Build history of the part. All positions in model axes, mm. Face numbers are marked on the shaded views. A direction names the side the tool comes from. Give positions to 0.01 mm unless a question says otherwise; leave off trailing zeros. Order: outer loops, then holes, each group sorted by start corner. A loop starts at its lowest first (then second) coordinate and runs counter-clockwise, first axis right, second up. Notation, with made-up numbers: (79.25, 81) - (104.25, 81) arc R15 cw to (104.25, 90) - close; hole circle Ø2 at (-9.75, 0). An arc over 180 degrees is marked (long way). Answer in a Markdown table with one row per item.
```python
from build123d import *

# Parameters (mm, degrees)
SKETCH_1_W               = 17.5
SKETCH_1_H               = 55
EXTRUDE_1_DEPTH          = 2
SKETCH_2_W               = 5
SKETCH_2_H               = 5
EXTRUDE_2_DEPTH          = 33
EXTRUDE_3_DEPTH          = 6.5
EXTRUDE_3_DEPTH_BACK     = 8.378522314
SKETCH_3_W               = 5
SKETCH_3_H               = 55
SKETCH_4_R               = 1.5
CUT_EXTRUDE_1_DEPTH      = 10
FILLET_1_R               = 10
SKETCH_5_R               = 4
CUT_EXTRUDE_2_DEPTH      = 12
EXTRUDE_START            = -14.878522
EXTRUDE_4_DEPTH          = 14.878522
SKETCH_7_W               = 4
SKETCH_7_H               = 2
SKETCH_7_W_2             = 2.3
SKETCH_7_H_2             = 5.8
EXTRUDE_5_DEPTH          = 42.173435595
SKETCH_9_R               = 2
CUT_EXTRUDE_15_DEPTH     = 39
CUT_EXTRUDE_START        = -6.3
CUT_EXTRUDE_16_OUTLINE_W = 24
CUT_EXTRUDE_16_OUTLINE_H = 9.8
CUT_EXTRUDE_16_DEPTH     = 6.3


# Read off the part's stored shape, not the designer's step: Вырез-Вытянуть16
with BuildPart() as part:
    # Эскиз1 → Бобышка-Вытянуть1 (new body)
    with BuildSketch(Plane(origin=(0, 0, 0), x_dir=(1, 0, 0), z_dir=(0, 1, 0))):
        with Locations((8.75, 27.5)):
            Rectangle(SKETCH_1_W, SKETCH_1_H)
    extrude(amount=EXTRUDE_1_DEPTH)

    # Эскиз2 → Бобышка-Вытянуть2 (add)
    with BuildSketch(Plane(origin=(0, 2, 0), x_dir=(1, 0, 0), z_dir=(0, 1, 0))):
        with Locations((2.5, 52.5)):
            Rectangle(SKETCH_2_W, SKETCH_2_H)
        with Locations((2.5, 2.5)):
            Rectangle(SKETCH_2_W, SKETCH_2_H)
    extrude(amount=EXTRUDE_2_DEPTH)

    # Эскиз3 → Бобышка-Вытянуть3 (add, two sides: drawn at the far end of the back side and taken through both)
    with BuildSketch(Plane(origin=(0, 35, 0), x_dir=(1, 0, 0), z_dir=(0, 1, 0)).offset(-EXTRUDE_3_DEPTH_BACK)):
        with Locations((2.5, 27.5)):
            Rectangle(SKETCH_3_W, SKETCH_3_H)
    extrude(amount=EXTRUDE_3_DEPTH + EXTRUDE_3_DEPTH_BACK)

    # Эскиз4 → Вырез-Вытянуть1 (cut)
    with BuildSketch(Plane(origin=(0, 2, 0), x_dir=(1, 0, 0), z_dir=(0, 1, 0))):
        with Locations(Location((11.449842766, 48, 0), (0, 0, 270))):
            Circle(SKETCH_4_R)
        with Locations(Location((11.449842766, 7, 0), (0, 0, 270))):
            Circle(SKETCH_4_R)
    extrude(amount=-CUT_EXTRUDE_1_DEPTH, mode=Mode.SUBTRACT)

    # Скругление1
    # the kernel refuses this fillet: 10 mm, written as the material it adds along each edge
    with BuildSketch(Plane(origin=(5, 2, -50), x_dir=(0, 0, 1), z_dir=(-1, 0, 0)), Plane(origin=(5, 2, 0), x_dir=(0, 1, 0), z_dir=(0, 0, -1))) as fillet_1_piece_1:
        with BuildLine():
            CenterArc((FILLET_1_R, FILLET_1_R), FILLET_1_R, 180, 90)
            Line((0, FILLET_1_R), (0, 0))
            Line((0, 0), (FILLET_1_R, 0))
        make_face()
    extrude(amount=5)
    with BuildSketch(Plane(origin=(5, 2, -55), x_dir=(0, 1, 0), z_dir=(0, 0, 1)), Plane(origin=(5, 2, -5), x_dir=(0, 0, -1), z_dir=(-1, 0, 0))) as fillet_1_piece_2:
        with BuildLine():
            CenterArc((FILLET_1_R, -FILLET_1_R), FILLET_1_R, 90, 90)
            Line((0, -FILLET_1_R), (0, 0))
            Line((0, 0), (FILLET_1_R, 0))
        make_face()
    extrude(amount=5)
    with BuildSketch(Plane(origin=(5, 2, -55), x_dir=(0, 1, 0), z_dir=(0, 0, 1))) as fillet_1_piece_3a_section:
        with BuildLine():
            CenterArc((FILLET_1_R, -FILLET_1_R), FILLET_1_R, 90, 90)
            Line((0, -FILLET_1_R), (0, 0))
            Line((0, 0), (FILLET_1_R, 0))
        make_face()
    fillet_1_piece_3a = extrude(amount=30, mode=Mode.PRIVATE)
    fillet_1_piece_3a = split(fillet_1_piece_3a, bisect_by=Plane(origin=(7.224830191, 4.283537978, -50), z_dir=(0, 0, 1)), keep=Keep.TOP, mode=Mode.PRIVATE)
    fillet_1_piece_3a = fillet_1_piece_3a - Plane(origin=(11.449842766, 4.283537978, -48), x_dir=(0, 0, 1), z_dir=(0, 1, 0)) * Cylinder(1.5, 100, mode=Mode.PRIVATE)
    with BuildSketch(Plane(origin=(30, 2, -50), x_dir=(0, 0, 1), z_dir=(-1, 0, 0))) as fillet_1_piece_3b_section:
        with BuildLine():
            CenterArc((FILLET_1_R, FILLET_1_R), FILLET_1_R, 180, 90)
            Line((0, FILLET_1_R), (0, 0))
            Line((0, 0), (FILLET_1_R, 0))
        make_face()
    fillet_1_piece_3b = extrude(amount=30, mode=Mode.PRIVATE)
    fillet_1_piece_3b = split(fillet_1_piece_3b, bisect_by=Plane(origin=(5, 2.276950555, -42.605283247), z_dir=(1, 0, 0)), keep=Keep.TOP, mode=Mode.PRIVATE)
    fillet_1_piece_3b = split(fillet_1_piece_3b, bisect_by=Plane(origin=(17.5, 2.276950555, -42.605283247), z_dir=(-1, 0, 0)), keep=Keep.TOP, mode=Mode.PRIVATE)
    fillet_1_piece_3b = fillet_1_piece_3b - Plane(origin=(11.449842766, 2.276950555, -48), x_dir=(0, 0, 1), z_dir=(0, 1, 0)) * Cylinder(1.5, 100, mode=Mode.PRIVATE)
    fillet_1_piece_3 = fillet_1_piece_3a & fillet_1_piece_3b
    add(fillet_1_piece_3)
    with BuildSketch(Plane(origin=(5, 2, 0), x_dir=(0, 1, 0), z_dir=(0, 0, -1))) as fillet_1_piece_4a_section:
        with BuildLine():
            CenterArc((FILLET_1_R, FILLET_1_R), FILLET_1_R, 180, 90)
            Line((0, FILLET_1_R), (0, 0))
            Line((0, 0), (FILLET_1_R, 0))
        make_face()
    fillet_1_piece_4a = extrude(amount=30, mode=Mode.PRIVATE)
    fillet_1_piece_4a = split(fillet_1_piece_4a, bisect_by=Plane(origin=(7.224831151, 4.283537771, -5), z_dir=(0, 0, -1)), keep=Keep.TOP, mode=Mode.PRIVATE)
    fillet_1_piece_4a = fillet_1_piece_4a - Plane(origin=(11.449842766, 4.283537771, -7), x_dir=(0, 0, 1), z_dir=(0, 1, 0)) * Cylinder(1.5, 100, mode=Mode.PRIVATE)
    with BuildSketch(Plane(origin=(30, 2, -5), x_dir=(0, 0, -1), z_dir=(-1, 0, 0))) as fillet_1_piece_4b_section:
        with BuildLine():
            CenterArc((FILLET_1_R, -FILLET_1_R), FILLET_1_R, 90, 90)
            Line((0, -FILLET_1_R), (0, 0))
            Line((0, 0), (FILLET_1_R, 0))
        make_face()
    fillet_1_piece_4b = extrude(amount=30, mode=Mode.PRIVATE)
    fillet_1_piece_4b = split(fillet_1_piece_4b, bisect_by=Plane(origin=(5, 2.276949142, -12.394716375), z_dir=(1, 0, 0)), keep=Keep.TOP, mode=Mode.PRIVATE)
    fillet_1_piece_4b = split(fillet_1_piece_4b, bisect_by=Plane(origin=(17.5, 2.276949142, -12.394716375), z_dir=(-1, 0, 0)), keep=Keep.TOP, mode=Mode.PRIVATE)
    fillet_1_piece_4b = fillet_1_piece_4b - Plane(origin=(11.449842766, 2.276949142, -7), x_dir=(0, 0, 1), z_dir=(0, 1, 0)) * Cylinder(1.5, 100, mode=Mode.PRIVATE)
    fillet_1_piece_4 = fillet_1_piece_4a & fillet_1_piece_4b
    add(fillet_1_piece_4)

    # Эскиз5 → Вырез-Вытянуть2 (cut)
    with BuildSketch(Plane(origin=(0, 2, 0), x_dir=(1, 0, 0), z_dir=(0, 1, 0))):
        with Locations((11.449842766, 48)):
            Circle(SKETCH_5_R)
        with Locations((11.449842766, 7)):
            Circle(SKETCH_5_R)
    extrude(amount=CUT_EXTRUDE_2_DEPTH, mode=Mode.SUBTRACT)

    # Эскиз6 → Бобышка-Вытянуть4 (add)
    with BuildSketch(Plane(origin=(0, 41.5, 0), x_dir=(1, 0, 0), z_dir=(0, 1, 0)).offset(EXTRUDE_START)):
        with BuildLine():
            Line((0, 4.85), (0, 6.15))
            Line((0, 6.15), (-1.92, 6.15))
            Line((-1.92, 6.15), (-2.88, 4.487231225))
            ThreePointArc((-2.88, 4.487231225), (-2.642083488, 3.599314712), (-1.754166975, 3.837231225))
            Line((-1.754166975, 3.837231225), (-1.16944465, 4.85))
            Line((-1.16944465, 4.85), (0, 4.85))
        make_face()
        with BuildLine():
            Line((0, 28.65), (0, 29.95))
            Line((0, 29.95), (-1.16944465, 29.95))
            Line((-1.16944465, 29.95), (-1.754166975, 30.962768775))
            ThreePointArc((-1.754166975, 30.962768775), (-2.642083488, 31.200685288), (-2.88, 30.312768775))
            Line((-2.88, 30.312768775), (-1.92, 28.65))
            Line((-1.92, 28.65), (0, 28.65))
        make_face()
    extrude(amount=EXTRUDE_4_DEPTH)

    # Эскиз7 → Бобышка-Вытянуть5 (add)
    with BuildSketch(Plane.XY):
        with Locations((9.3, 40.5)):
            Rectangle(SKETCH_7_W, SKETCH_7_H)
        with Locations((6.15, 40.5)):
            Rectangle(SKETCH_7_W_2, SKETCH_7_H)
        with Locations((9.3, 36.6)):
            Rectangle(SKETCH_7_W, SKETCH_7_H_2)
        Polygon((7.3, 33.7), (5, 33.7), (5, 31.7), (11.3, 31.7), (11.3, 33.7), align=None)
    extrude(amount=-EXTRUDE_5_DEPTH)

    # Эскиз9 → Вырез-Вытянуть15 (cut)
    with BuildSketch(Plane(origin=(11.3, 0, 0), x_dir=(0, 0, -1), z_dir=(1, 0, 0))):
        with Locations((37, 36.5)):
            Circle(SKETCH_9_R)
        with Locations((5, 36.5)):
            Circle(SKETCH_9_R)
    extrude(amount=-CUT_EXTRUDE_15_DEPTH, mode=Mode.SUBTRACT)

    # Вырез-Вытянуть16 outline → Вырез-Вытянуть16 (cut)
    with BuildSketch(Plane(origin=(11.3, 0, 0), x_dir=(0, 0, -1), z_dir=(1, 0, 0)).offset(CUT_EXTRUDE_START)):
        with Locations((21, 36.6)):
            Rectangle(CUT_EXTRUDE_16_OUTLINE_W, CUT_EXTRUDE_16_OUTLINE_H)
    extrude(amount=CUT_EXTRUDE_16_DEPTH, mode=Mode.SUBTRACT)


solid = part.part
```
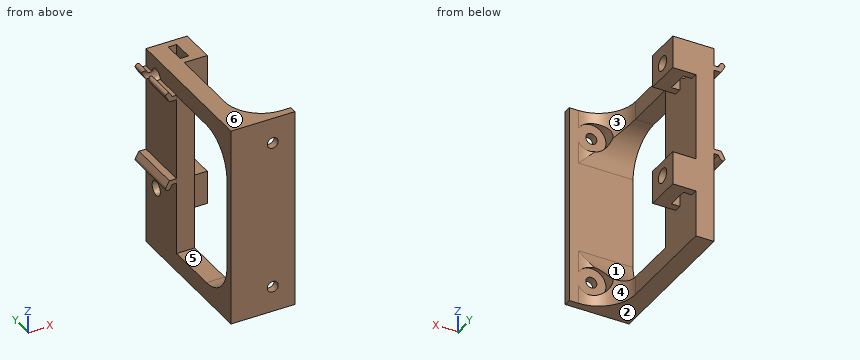
1. Cut at C-C on x = 2. Write the cut outline in (y, z).
Check result:
| item | result |
|---|---|
| outline | (0, -55) - (41.5, -55) - (41.5, 0) - (0, 0) - close; hole (2, -40) arc R10 ccw to (12, -50) - (26.62, -50) - (26.62, -5) - (12, -5) arc R10 ccw to (2, -15) - close; hole circle Ø4 at (36.5, -37); hole circle Ø4 at (36.5, -5) |
2. Cut at B-B on z = -25.5. Write the cut outline in (x, y).
Check result:
| item | result |
|---|---|
| outline | (0, 0) - (17.5, 0) - (17.5, 2) - (0, 2) - close; (0, 26.62) - (5, 26.62) - (5, 41.5) - (0, 41.5) - close |
3. Drop flat-ended pins along their axis: P1, Ø2, axis at x = -1.5, y = 31, coming from the -Z side; P2, Ø4, axis at y = 28, z = -16.5, coming from the +X side; P3, Ø3, axis at y = 35.5, z = -35.5, coming from the +X side; P4, Ø4, axis at y = 7, z = -45, coming from the +X side. Give the stop position or say it passes through.
Check result:
| item | result |
|---|---|
| P1 | stops at z = -31.29 |
| P2 | stops at x = 5 |
| P3 | stops at x = 11.3 |
| P4 | passes through |
4. Which spindle directions (+Z, -Z, +X, -X, +Y, -Y) get a long thin tool onto all of the face, cutting with end or side? Do the marked faces 1 and 2. Say none if no direction does.
Check result:
| item | result |
|---|---|
| face 1 | +X, -X |
| face 2 | -Z, +X, -X, +Y, -Y |
5. Probe line 1 (Y direction, x = 9.3, z = -37); line 2 (Y direction, x = -0.5, z = -5); line 3 (Y direction, x = 1, z = -14.5). List the from-to ranges inside material, lowest first.
Check result:
| item | result |
|---|---|
| line 1 | y = 0 to 2, 31.7 to 34.5, 38.5 to 41.5 |
| line 2 | y = 26.62 to 34.5, 38.5 to 41.5 |
| line 3 | y = 0 to 2.01, 26.62 to 41.5 |
6. Cut at D-D on y = 36.5. Count the separate pieces of the cut face and the enclosed holes in it, and give its area (3 significant figures).
Check result:
| item | result |
|---|---|
| separate pieces | 7 |
| enclosed holes | 0 |
| area | 280 mm² |
7. Two-plate mould, pull along Y, no slides. Class the marked faces 3, 4, 5 and 6: +Y half, -Y half, draft (parallel to the pull), parting line (faces both ways), or undercut.
Check result:
| item | result |
|---|---|
| face 3 | undercut |
| face 4 | +Y half |
| face 5 | undercut |
| face 6 | draft |
8. Cut at A-A on y = 15.5. Write the cut outline in (x, z).
Check result:
| item | result |
|---|---|
| outline | (0, -55) - (5, -55) - (5, -50) - (0, -50) - close; (0, -5) - (5, -5) - (5, 0) - (0, 0) - close |
